```python
from build123d import *

# Parameters (mm, degrees)
FILLET1_R          = 3
SKETCH2_R          = 1.2
CUT_EXTRUDE1_DEPTH = 10


with BuildPart() as part:
    # Sketch1 one side → Revolve1 (revolve)
    with BuildSketch(Plane.XY, mode=Mode.PRIVATE) as revolve1_sk:
        with BuildLine():
            Line((6.5, 8.5), (0, 8.5))
            Line((0, 8.5), (0, -7))
            ThreePointArc((0, -7), (3.456192986, -5.967326651), (5.779332516, -3.207850808))
            Line((5.779332516, -3.207850808), (5.996722799, -3.207850808))
            ThreePointArc((5.996722799, -3.207850808), (6.15577987, -1.598658708), (5.9126982, 0))
            Line((5.9126982, 0), (13, 0))
            Line((13, 0), (13, 2))
            Line((13, 2), (9.5, 2))
            Line((9.5, 2), (6.5, 8.5))
        make_face()
    revolve(revolve1_sk.sketch.rotate(Axis((0, 8.5, 0), (0, -1, 0)), 90), axis=Axis((0, 8.5, 0), (0, -1, 0)))

    # Fillet1
    fillet1_edges = [part.edges().sort_by_distance(p)[0] for p in [
        (0, 0, -5.9126982),
    ]]
    fillet(fillet1_edges, radius=FILLET1_R)

    # Sketch2 → Cut-Extrude1 (cut)
    with BuildSketch(Plane.XZ):
        with Locations(Location((0, 11, 0), (0, 0, 270))):
            Circle(SKETCH2_R)
        with Locations(Location((9.526279442, -5.5, 0), (0, 0, 270))):
            Circle(SKETCH2_R)
        with Locations(Location((-9.526279442, -5.5, 0), (0, 0, 270))):
            Circle(SKETCH2_R)
    extrude(amount=-CUT_EXTRUDE1_DEPTH, mode=Mode.SUBTRACT)


solid = part.part
```
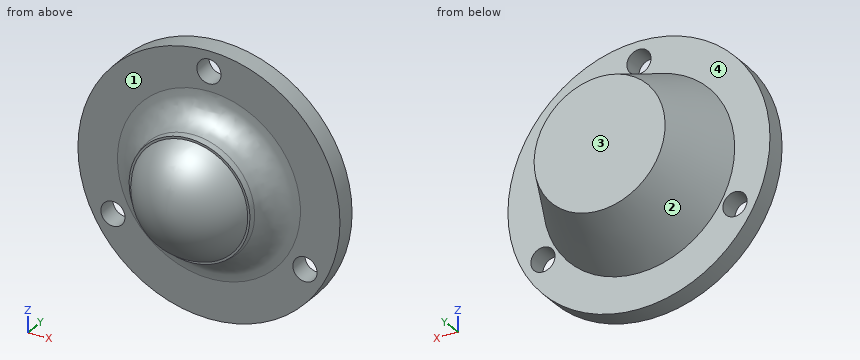
Geometry check sheet. Reference: the model listing, model coordinates, mm. Face numbers are marked on the shaded views. A direction names the side the tool comes from. Coordinates: 2 decimals unless noted, no trailing zeros. Order: outer loops, then holes, each group sorted by start corner. A loop starts at its lowest first (then second) coordinate and runs counter-clockwise, first axis right, second up.
Item 1: Mould release check, pull along X, two halves, no side actions. Record for the marked faces 1 and 2: released by +X, released by -X, zero draft, split by the parting line, or undercut.
Item 2: Section check B-B (z = -5). Count the separate pieces of the cut face and the enclosed holes in it, plus the area to 3 significant figures.
Item 3: Tool access check on the marked faces 3 and 4. Record the directions out of +Z, -Z, +X, -X, +Y, -Y that give a thin tool (end or side, any length) a straight path to the whole face; none if there is none.
Item 4: Section check C-C (y = -6). Enter the section's corners in (x, z), plus the area to 3 significant figures.
Item 5: Scan lines: line 1 along X through (y, z) = (1.35, -5.5); line 2 along Y through (x, z) = (-11.25, 4.5); line 3 along X through (y, z) = (1.45, 11). Record each from-to range of solid material in increasing order.
Item 6: Depth check by flat-ended pin: pin 1 (8 mm diameter, centred on x = 3.5, z = 3.5, fed in from -Y); pin 2 (1 mm diameter, centred on y = 0, z = 4.5, fed in from -X); pin 3 (10 mm diameter, centred on x = 4.5, z = -5.5, fed in from -Y). Enter the tip coordinate at first touch or a pass-through.
Item 7: Section check D-D (y = -4). Enter the section's corners in (x, z), plus the area to 3 significant figures.
Item 8: Section check A-A (z = 11.5). Enter the section's corners in (x, y).
Check sheet entries:
1. face 1: zero draft
1. face 2: split by the parting line
2. separate pieces: 3
2. enclosed holes: 0
2. area: 153 mm2
3. face 3: +Z, -Z, +X, -X, +Y
3. face 4: +Y
4. outline: circle Ø6.81 at (0, 0)
4. area: 36.4 mm2
5. line 1: x = -11.78 to -10.73, -8.33 to 8.33, 10.73 to 11.78
5. line 2: y = 0 to 2
5. line 3: x = -6.93 to -1.2, 1.2 to 6.93
6. pin 1: stops at y = -6.93
6. pin 2: stops at x = -12.37
6. pin 3: stops at y = -6.64
7. outline: circle Ø10.73 at (0, 0)
7. area: 90.5 mm2
8. outline: (-6.06, 0) - (-1.09, 0) - (-1.09, 2) - (-6.06, 2) - close; (1.09, 0) - (6.06, 0) - (6.06, 2) - (1.09, 2) - close
